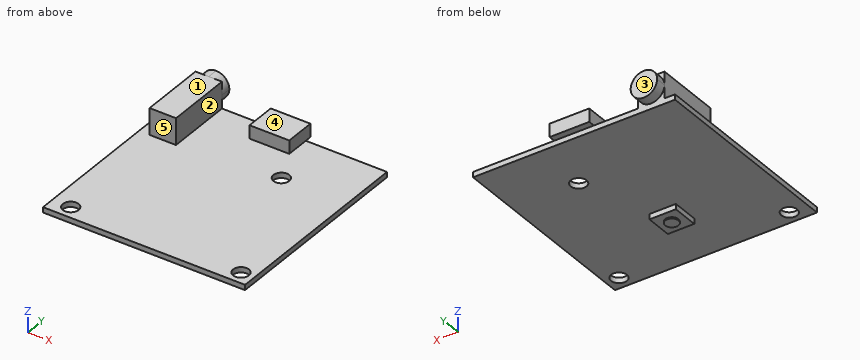
```python
from build123d import *

# Parameters (mm, degrees)
F0_W      = 38.2
F0_H      = 38.6
F0_R      = 1.5
F1_DEPTH  = 1
F2_W      = 7.5
F2_H      = 4.5
F2_H_2    = 1.25
F3_DEPTH  = 2.5
F4_W      = 5
F4_H      = 5
F5_DEPTH  = 1
F6_R      = 1.25
F7_DEPTH  = 0.25
F8_W      = 5
F8_H      = 12.5
F9_DEPTH  = 5
F11_DEPTH = 2


with BuildPart() as f1:
    # F0 (on Top) → F1 (new body)
    with BuildSketch(Plane.XY):
        Rectangle(F0_W, F0_H)
        with Locations((-15.6, -16.8)):
            Circle(F0_R, mode=Mode.SUBTRACT)
        with Locations((16.6, -16.8)):
            Circle(F0_R, mode=Mode.SUBTRACT)
        with Locations((6.6, 8.55)):
            Circle(F0_R, mode=Mode.SUBTRACT)
    extrude(amount=F1_DEPTH)

    # F2 (on face) → F3 (join)
    with BuildSketch(Plane.XY.offset(1)):
        with Locations((0, 17.05)):
            Rectangle(F2_W, F2_H)
        with Locations((0, 19.925)):
            Rectangle(F2_W, F2_H_2)
    extrude(amount=F3_DEPTH)

    # F4 (on face) → F5 (join)
    with BuildSketch(Plane(origin=(0, 0, 0), x_dir=(1, 0, 0), z_dir=(0, 0, -1))):
        with Locations((0, 7.3)):
            Rectangle(F4_W, F4_H)
    extrude(amount=F5_DEPTH)

    # F6 (on face) → F7 (join)
    with BuildSketch(Plane(origin=(0, 0, -1), x_dir=(1, 0, 0), z_dir=(0, 0, -1))):
        with Locations((0, 7.3)):
            Circle(F6_R)
    extrude(amount=F7_DEPTH)

    # F8 (on face) → F9 (join)
    with BuildSketch(Plane.XY.offset(1)):
        with Locations((-14.6, 13.05)):
            Rectangle(F8_W, F8_H)
    extrude(amount=F9_DEPTH)

    # F10 (on face) → F11 (join)
    with BuildSketch(Plane(origin=(0, 19.3, 0), x_dir=(-1, 0, 0), z_dir=(0, 1, 0))):
        with BuildLine():
            ThreePointArc((12.1, 3.5), (14.6, 1), (17.1, 3.5))
            ThreePointArc((17.1, 3.5), (16.367767, 5.267767), (14.6, 6))
            ThreePointArc((14.6, 6), (12.832233, 5.267767), (12.1, 3.5))
        make_face()
    extrude(amount=F11_DEPTH)


solid = f1.part
```
Could you check a few things on this model? Use its own coordinates, in mm. Face numbers are marked on the shaded views. A direction names the side the tool comes from. Coordinates: 2 decimals unless noted, no trailing zeros. Write each loop counter-clockwise with the first axis right and the second up, starting at its lowest first coordinate (ties: lowest second). Pieces come first, ordered by that corner, then holes. Notation, with made-up numbers: (65.25, 39.5) - (97.25, 39.5) arc R18 ccw to (97.25, 62.5) - close; hole circle Ø7 at (7.5, 49). An arc over 180 degrees is marked (long way). Use a Markdown table: item, result.
Q1. Imagine slicing it at C-C (x = 6.6). List the corners of the cut face in (y, z) for me.
Geometry check:
| item | result |
|---|---|
| outline | (-19.3, 0) - (7.05, 0) - (7.05, 1) - (-19.3, 1) - close; (10.05, 0) - (19.3, 0) - (19.3, 1) - (10.05, 1) - close |
Q2. Which directions (+Z, -Z, +X, -X, +Y, -Y) give clear straight access to the entire face, cutting with the end or side of a thin tool? Please do the marked faces 3, 4 and 5.
Geometry check:
| item | result |
|---|---|
| face 3 | +Z, -Z, +X, -X, +Y |
| face 4 | +Z, +X, +Y, -Y |
| face 5 | +Z, +X, -X, -Y |
Q3. Imagine slicing it at B-B (z = 1.5). List the corners of the cut face in (x, y) for me, and give its area (3 significant figures).
Geometry check:
| item | result |
|---|---|
| outline | (-17.1, 6.8) - (-12.1, 6.8) - (-12.1, 19.3) - (-13.1, 19.3) - (-13.1, 21.3) - (-16.1, 21.3) - (-16.1, 19.3) - (-17.1, 19.3) - close; (-3.75, 14.8) - (3.75, 14.8) - (3.75, 20.55) - (-3.75, 20.55) - close |
| area | 112 mm2 |
Q4. I'm going to push flat-ended pins straight in: pin 1 Ø1.7 at (x, y) = (0, 18) entering from +Z; pin 2 Ø3 at (x, z) = (1, 2) entering from +Y; pin 3 Ø4 at (x, y) = (-12, 2) entering from +Z. Where does each tip first touch, or does it pass through?
Geometry check:
| item | result |
|---|---|
| pin 1 | stops at z = 3.5 |
| pin 2 | stops at y = 20.55 |
| pin 3 | stops at z = 1 |
Q5. Please list where these lines run through material, in increasing order: L1, parallel to Y at x = -15.6, z = 0.4; L2, parallel to Y at x = 6.6, z = 0.8; L3, parallel to Z at x = 10.5, y = 9.5.
Geometry check:
| item | result |
|---|---|
| L1 | y = -19.3 to -18.3, -15.3 to 19.3 |
| L2 | y = -19.3 to 7.05, 10.05 to 19.3 |
| L3 | z = 0 to 1 |
Q6. Thinking about a two-plate mould opening in Z: for the marked faces 1 and 2, which applies, +Z half, -Z half, draft (parallel to the pull), parting line (faces both ways), or undercut?
Geometry check:
| item | result |
|---|---|
| face 1 | +Z half |
| face 2 | draft |
Q7. Imagine slicing it at A-A (y = 11). List the corners of the cut face in (x, z) for me, and give its area (3 significant figures).
Geometry check:
| item | result |
|---|---|
| outline | (-19.1, 0) - (19.1, 0) - (19.1, 1) - (-12.1, 1) - (-12.1, 6) - (-17.1, 6) - (-17.1, 1) - (-19.1, 1) - close |
| area | 63.2 mm2 |
Q8. Imagine slicing it at D-D (x = 0). List the corners of the cut face in (y, z) for me.
Geometry check:
| item | result |
|---|---|
| outline | (-19.3, 0) - (-9.8, 0) - (-9.8, -1) - (-8.55, -1) - (-8.55, -1.25) - (-6.05, -1.25) - (-6.05, -1) - (-4.8, -1) - (-4.8, 0) - (19.3, 0) - (19.3, 1) - (20.55, 1) - (20.55, 3.5) - (14.8, 3.5) - (14.8, 1) - (-19.3, 1) - close |
